Work out the finished part from the listing and answer in its coordinate system (mm). Give positions to 0.01 mm unless a question says otherwise; leave off trailing zeros. Write each loop counter-clockwise with the first axis right and the second up, starting at its lowest first coordinate (ties: lowest second). Pieces come first, ordered by that corner, then holes. Notation, with made-up numbers: (24.25, 88.5) - (54.25, 88.5) arc R25 ccw to (54.25, 101.5) - close; hole circle Ø1 at (9, 62.25). An arc over 180 degrees is marked (long way). Write each question's results on one line, items separated by ' | '. Start each with the question number.
from build123d import *

# Parameters (mm, degrees)
F1_DEPTH = 800


with BuildPart() as f1:
    # F0 (on Front) → F1 (new body)
    with BuildSketch(Plane.XZ):
        with BuildLine():
            ThreePointArc((-10, -29.030345), (-10.133975, -29.530345), (-10.5, -29.89637))
            Line((-10.5, -29.89637), (-22, -36.535898))
            ThreePointArc((-22, -36.535898), (-23.464102, -42), (-18, -43.464102))
            Line((-18, -43.464102), (-11.5, -39.711325))
            ThreePointArc((-11.5, -39.711325), (-10.5, -39.711325), (-10, -40.57735))
            Line((-10, -40.57735), (-10, -49))
            ThreePointArc((-10, -49), (-9.707107, -49.707107), (-9, -50))
            Line((-9, -50), (-5, -50))
            ThreePointArc((-5, -50), (-4.292893, -50.292893), (-4, -51))
            Line((-4, -51), (-4, -54))
            Line((-4, -54), (-3, -55))
            Line((-3, -55), (-4, -56))
            Line((-4, -56), (-4, -59))
            ThreePointArc((-4, -59), (-3.707107, -59.707107), (-3, -60))
            Line((-3, -60), (0, -60))
            Line((0, -60), (0, -15))
            Line((0, -15), (-3, -15))
            ThreePointArc((-3, -15), (-3.707107, -15.292893), (-4, -16))
            Line((-4, -16), (-4, -19))
            Line((-4, -19), (-3, -20))
            Line((-3, -20), (-4, -21))
            Line((-4, -21), (-4, -24))
            ThreePointArc((-4, -24), (-4.292893, -24.707107), (-5, -25))
            Line((-5, -25), (-9, -25))
            ThreePointArc((-9, -25), (-9.707107, -25.292893), (-10, -26))
            Line((-10, -26), (-10, -29.030345))
        make_face()
    extrude(amount=-F1_DEPTH)


solid = f1.part
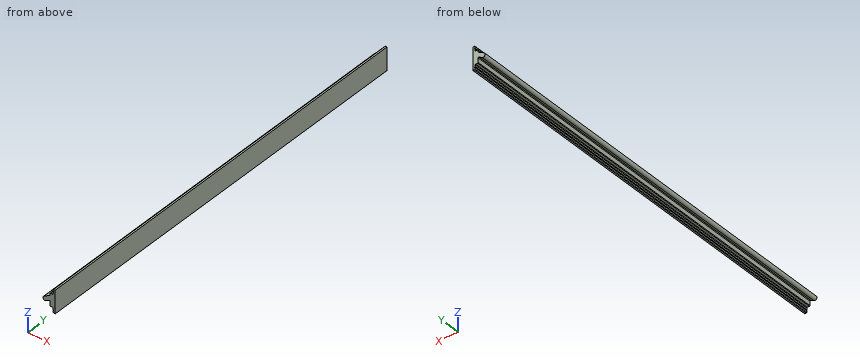
Q1. Consider L1, parallel to X at y = 693, z = -43.5; L2, parallel to X at y = 544.5, z = -41; L3, parallel to X at y = 599.5, z = -28.5. Determine where each line is inside the solid, lowest interval first.
Q2. A cutting plane is placed at A-A, the plane y = 503. Write down the section's boundary in (x, z).
Q3. Given pin 1 (1.2 mm diameter, centred on x = -8, y = 521, fed in from -Z); pin 2 (2.5 mm diameter, centred on y = 338.5, z = -22.5, fed in from -X); pin 3 (4.5 mm diameter, centred on x = -7.5, y = 402, fed in from +Z), each flat-ended and moving along its own axis, determine where each tip first touches the part or whether it passes through.
Result:
1) L1: x = -21.94 to -18.06, -10 to 0 | L2: x = -23.87 to -13.73, -10 to 0 | L3: x = -10 to 0
2) outline: (-22, -36.54) arc R4 ccw to (-18, -43.46) - (-11.5, -39.71) arc R1 cw to (-10, -40.58) - (-10, -49) arc R1 ccw to (-9, -50) - (-5, -50) arc R1 cw to (-4, -51) - (-4, -54) - (-3, -55) - (-4, -56) - (-4, -59) arc R1 ccw to (-3, -60) - (0, -60) - (0, -15) - (-3, -15) arc R1 ccw to (-4, -16) - (-4, -19) - (-3, -20) - (-4, -21) - (-4, -24) arc R1 cw to (-5, -25) - (-9, -25) arc R1 ccw to (-10, -26) - (-10, -29.03) arc R1 cw to (-10.5, -29.9) - close
3) pin 1: stops at z = -50 | pin 2: stops at x = -4 | pin 3: stops at z = -25
